Autodesk Inventor part; units mm, degrees
ref_plane "YZ Plane" through (0, 0, 0) normal (1, 0, 0) x (0, 1, 0)
ref_plane "XZ Plane" through (0, 0, 0) normal (0, 1, 0) x (-1, 0, 0)
ref_plane "XY Plane" through (0, 0, 0) normal (0, 0, 1) x (1, 0, 0)
sketch "Sketch1" plane through (0, 0, 0) normal (0, 0, 1) x (1, 0, 0)
  line L0 (-490, 50) -> (490, 50)
  line L1 (490, 50) -> (490, 0)
  line L2 (490, 0) -> (-490, 0)
  line L3 (-490, 0) -> (-490, 50)
  point P0 (0, 0)
  point P1 (0, 0)
  dimension "d0" = 980
  dimension "d1" = 50
extrude "Plate1" add sketch "Sketch1" along normal blind 2
sketch "Sketch2" plane through (490, 2, 0) normal (0, -1, 0) x (1, 0, 0)
  line L0 (-980, 0) -> (0, 0)
  line L1 (0, 0) -> (0, 20)
  line L2 (0, 20) -> (-980, 20)
  line L3 (-980, 20) -> (-980, 0)
edge flange "Flange1" height 20 angle 90 thickness 2 bend radius 2.75 thickness toward (0, -1, 0) relief tear relief width 2 relief depth 1 edges at (0, 0, 2) wall of the first edge with corners at (-490, 2, 0) (490, 2, 0) (490, 2, 20) (-490, 2, 20)
bend "Bend1"
corner "Corner1"
sketch "Sketch5" plane through (0, 0, 0) normal (0, 0, -1) x (-1, 0, 0)
  line L0 (490, 50) -> (-490, 50)
  line L1 (490, 0) -> (-490, 0)
  circle A0 centre (0, 50) radius 30
  line L2 (-490, 0) -> (-490, 50)
  line L3 (490, 0) -> (490, 50)
  circle A1 centre (-490, 50) radius 30
  circle A2 centre (490, 50) radius 30
  line L4 (-241, 50) -> (-239, 50)
  line L5 (-239, 50) -> (-239, 19)
  line L6 (-239, 19) -> (-241, 19)
  line L7 (-241, 19) -> (-241, 50)
  line L8 (239, 50) -> (241, 50)
  line L9 (241, 50) -> (241, 19)
  line L10 (241, 19) -> (239, 19)
  line L11 (239, 19) -> (239, 50)
  line L12 (0, 50) -> (0, 0) construction
  point P0 (240, 19)
  point P1 (-240, 19)
  point P2 (-490, 20)
  point P3 (-460, 50)
  point P4 (-30, 50)
  point P5 (30, 50)
  point P6 (460, 50)
  point P7 (490, 20)
  dimension "d33" = 60
  dimension "d34" = 2
  dimension "d35" = 31
  dimension "d36" = 480
extrude "Extrusion1" cut sketch "Sketch5" against normal through all contours L9 L10 L11 L0 | L0 L3 A2 | A0 L0 | L5 L6 L7 L0 | L2 L0 A1 picked at (470.2507, 47.7748) picked at (6.5355, 34.7298) picked at (-470.2507, 47.7748)
sketch "Sketch7" plane through (0, 0, 2) normal (0, 0, 1) x (1, 0, 0)
  line L0 (468.7934, 20.88) -> (468.7934, 8.88) construction
  line L1 (468.7934, 8.88) -> (280.354, 8.88) construction
  line L2 (280.354, 8.88) -> (280.354, 20.88) construction
  line L3 (280.354, 20.88) -> (468.7934, 20.88) construction
  line L4 (-239, 50) -> (-30, 50)
  point P0 (0, 0)
  point P1 (-1, 50)
  point P2 (1, 50)
  dimension "d30" = 12
mark "Mark1"
equation "\"d1\" = Стрингер_7"
equation "\"d2\" = Thickness"
equation "\"d3\" = BendReliefWidth"
equation "\"d4\" = BendReliefDepth"
equation "\"d5\" = MinimumRemnant"
equation "\"d6\" = TransitionRadius"
equation "\"d9\" = BendRadius"
equation "\"d10\" = CornerReliefSize"
equation "\"d11\" = GapSize"
equation "\"d12\" = JacobiRadiusSize"
equation "\"BendReliefWidth\" = Thickness"
equation "\"BendReliefDepth\" = 0.5 * Thickness"
equation "\"CornerReliefSize\" = 4 * Thickness"
equation "\"MinimumRemnant\" = 2 * Thickness"
equation "\"TransitionRadius\" = BendRadius"
equation "\"JacobiRadiusSize\" = BendRadius"
equation "\"GapSize\" = Thickness"
equation "\"Стрингер_7\" = 50"
properties part number "MSC 504 stringer board belly" material "Stainless Steel"
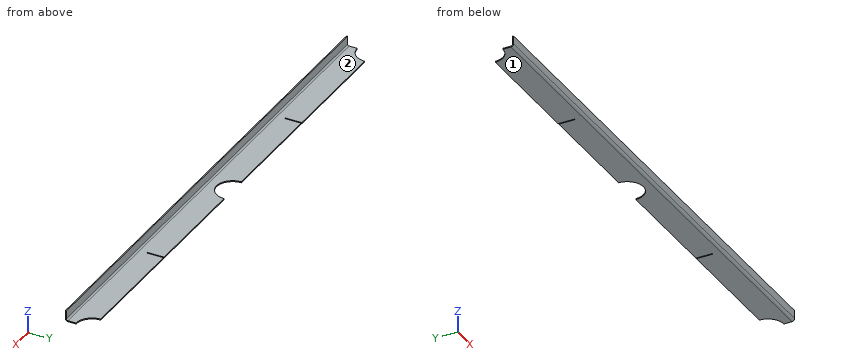
Part model, mm, in its own coordinate system. Face numbers are marked on the shaded views. Coordinates: 2 decimals unless noted, no trailing zeros. Write each loop counter-clockwise with the first axis right and the second up, starting at its lowest first coordinate (ties: lowest second). Pieces come first, ordered by that corner, then holes.
Item 1: Slice it at A-A (x = 0). Write the cut outline in (y, z), and give its area (3 significant figures).
Item 2: Slice it at C-C (z = 11.75). Write the cut outline in (x, y).
Item 3: Pin check, flat tips, straight feed: pin 1 (13.5 mm diameter, centred on x = 126, y = 35, fed in from +Z); pin 2 (1 mm diameter, centred on x = -240, z = 1, fed in from +Y); pin 3 (12 mm diameter, centred on x = -317, z = 12.5, fed in from +Y). Stop position of each tip, or through.
Item 4: Probe line 1 (Z direction, x = -364, y = 10); line 2 (Z direction, x = -184.5, y = 4). List the from-to ranges inside material, lowest first.
Item 5: Slice it at B-B (y = 39). Write the cut outline in (x, z).
Item 6: Mould opens along Z. For the marked faces 1 and 2 say: released by +Z, released by -Z, zero draft, split by the parting line, or undercut.
Results found:
1. outline: (0, 4.75) arc R4.75 ccw to (4.75, 0) - (20, 0) - (20, 2) - (4.75, 2) arc R2.75 cw to (2, 4.75) - (2, 20) - (0, 20) - close
1. area: 72.8 mm2
2. outline: (-490, 0) - (490, 0) - (490, 2) - (-490, 2) - close
3. pin 1: stops at z = 2
3. pin 2: stops at y = 19
3. pin 3: stops at y = 2
4. line 1: z = 0 to 2
4. line 2: z = 0.06 to 2.1
5. outline: (-462.09, 0) - (-241, 0) - (-241, 2) - (-462.09, 2) - close; (-239, 0) - (-27.91, 0) - (-27.91, 2) - (-239, 2) - close; (27.91, 0) - (239, 0) - (239, 2) - (27.91, 2) - close; (241, 0) - (462.09, 0) - (462.09, 2) - (241, 2) - close
6. face 1: released by -Z
6. face 2: released by +Z
